```python
from build123d import *

# Parameters (mm, degrees)
EXTRUDE_1_DEPTH = 14


with BuildPart() as part:
    # Эскиз1 → Бобышка-Вытянуть1 (new body)
    with BuildSketch(Plane(origin=(0, 0, 0), x_dir=(1, 0, 0), z_dir=(0, 1, 0))):
        Polygon((4.041451884, 0), (2.020725942, 3.5), (-2.020725942, 3.5), (-4.041451884, 0), (-2.020725942, -3.5), (2.020725942, -3.5), align=None)
    extrude(amount=EXTRUDE_1_DEPTH)

    # Эскиз2 → Отверстие обработанное метчиком M3x0.51 (revolve, cut)
    with BuildSketch(Plane(origin=(0, 14, 0), x_dir=(0, 0, 1), z_dir=(1, 0, 0))):
        Polygon((0, 0), (0, 14), (1.6, 14), (1.25, 13.754927362), (1.25, 0.245072638), (1.6, 0), align=None)
    revolve(axis=Axis((0, 20.35, 0), (0, -1, 0)), mode=Mode.SUBTRACT)


solid = part.part
```
For this review, take the finished solid that the model builds, in its own axes (mm). Round coordinates to 2 decimals unless told otherwise and drop trailing zeros. Loops run counter-clockwise (first coordinate to the right, second up) from the corner with the lowest first, then second, coordinate; pieces in that order, holes last.
(1) We need section D-D (x = 2.75). Give the boundary of the cut face in (y, z).
Returned:
outline: (0, -2.24) - (14, -2.24) - (14, 2.24) - (0, 2.24) - close
(2) Mouldability with a two-part tool opening along X and no side actions: class faces 1 (the flat face through (3, 6.9, 1.8)), 2 (the flat face through (-3, 6.9, -1.8)), 3 (the cylindrical face through (1.22, 7.09, -0.27)), 4 (the flat face through (0, 7, 3.5)) as released by +X, released by -X, zero draft, split by the parting line, or undercut.
Returned:
face 1: released by +X
face 2: released by -X
face 3: undercut
face 4: zero draft
(3) We need section B-B (y = 3). Give the boundary of the cut face in (x, z), plus the area to 3 significant figures.
Returned:
outline: (-4.04, 0) - (-2.02, -3.5) - (2.02, -3.5) - (4.04, 0) - (2.02, 3.5) - (-2.02, 3.5) - close; hole circle Ø2.5 at (0, 0)
area: 37.5 mm2
(4) We need section A-A (x = 0). Give the boundary of the cut face in (y, z), plus the area to 3 significant figures.
Returned:
outline: (0, -3.5) - (14, -3.5) - (14, -1.6) - (13.75, -1.25) - (0.25, -1.25) - (0, -1.6) - close; (0, 1.6) - (0.25, 1.25) - (13.75, 1.25) - (14, 1.6) - (14, 3.5) - (0, 3.5) - close
area: 62.8 mm2
(5) Wall thickness on line 1 along Z through (x, y) = (0, 7.5); line 2 along X through (y, z) = (10, -0.25); line 3 along X through (y, z) = (2.75, -0.75): over which ranges is each line inside the solid? List them lowest first.
Returned:
line 1: z = -3.5 to -1.25, 1.25 to 3.5
line 2: x = -3.9 to -1.22, 1.22 to 3.9
line 3: x = -3.61 to -1, 1 to 3.61
(6) We need section C-C (z = 1.75). Give the boundary of the cut face in (x, y).
Returned:
outline: (-3.03, 0) - (3.03, 0) - (3.03, 14) - (-3.03, 14) - close
(7) Clearance check with flat-ended pins moving along their axes: P1, Ø3, axis at x = 0, z = 0, coming from the -Y side; P2, Ø1.5, axis at y = 10, z = 2.5, coming from the -X side; P3, Ø1, axis at y = 10, z = 2, coming from the +X side. State where each tip first meets the part, or that it passes through.
Returned:
P1: stops at y = 0.07
P2: stops at x = -3.03
P3: stops at x = 3.18
